Geometry check sheet. Reference: the model listing, model coordinates, mm. A direction names the side the tool comes from. Round coordinates to 2 decimals unless told otherwise and drop trailing zeros. Loops run counter-clockwise (first coordinate to the right, second up) from the corner with the lowest first, then second, coordinate; pieces in that order, holes last. Notation, with made-up numbers: (-15, 35) -> (30, 35) arc R35 ccw to (30, 68) -> close; hole circle Ø4 at (63, 46.5). An arc over 180 degrees is marked (long way). Use a Markdown table: item, result. Add a question column.
Q1. Gauge pin test, flat ends, axial feed: P1, Ø5, axis at x = -1, y = 3.5, coming from the +Z side; P2, Ø1, axis at y = 23, z = 2, coming from the -X side; P3, Ø1.5, axis at y = -12.5, z = 1, coming from the -X side; P4, Ø21, axis at x = 0, y = 0, coming from the +Z side. Record the tip position at first contact, or that the pin passes through.
Q2. Release check for a two-part mould opening along Y. For faces 1 (the face through (-40.786, 1.077, 0.056)), 2 (the face through (-7, 0, -4)), 3 (the face through (-3, -6, -2)) record: released by +Y, released by -Y, zero draft, split by the parting line, or undercut.
Q3. Sectioned sample at A-A, the plane x = 0. Enter the section's corners in (y, z), then the cut area to 3 significant figures.
Q4. Set-up check for faces 4 (the face through (-8.25, -2.6, 0.96)), 5 (the face through (35.252, -0.296, -0.056)): record each of +Z, -Z, +X, -X, +Y, -Y from which the full face is reachable in a straight line by a thin tool's end or side.
Q5. Sectioned sample at B-B, the plane z = -3. Enter the section's corners in (x, y).
Q6. Material ranges on L1, parallel to Y at x = 0, z = -3.45; L2, parallel to Y at x = 20, z = -3; L3, parallel to Y at x = -4.5, z = -2.5, recorded low to high.
Q7. Sectioned sample at C-C, the plane z = 2.25. Enter the section's corners in (x, y), then the cut area to 3 significant figures.
```python
from build123d import *

# Parameters (mm, degrees)
SKETCH_1_R          = 40.8
EXTRUDE_1_DEPTH     = 4
SKETCH_3_R          = 3.15
CUT_EXTRUDE_1_DEPTH = 10
EXTRUDE_START       = -8
EXTRUDE_3_DEPTH     = 8
SKETCH_6_R          = 21
CUT_EXTRUDE_2_DEPTH = 10
SKETCH_7_R          = 0.5
CUT_EXTRUDE_3_DEPTH = 10


with BuildPart() as part:
    # 草图1 → 凸台-拉伸1 (new, symmetric)
    with BuildSketch(Plane.XY):
        Circle(SKETCH_1_R)
    extrude(amount=EXTRUDE_1_DEPTH, both=True)

    # 草图2 → 切除-旋转2 (revolve, cut)
    with BuildSketch(Plane(origin=(0, 0, 0), x_dir=(1, 0, 0), z_dir=(0, 1, 0)), mode=Mode.PRIVATE) as cut_revolve_2_sk:
        Polygon((0, 4), (0, -4), (8.65, -4), (8.65, 2), (6.5, 2), (6.5, 4), align=None)
    revolve(cut_revolve_2_sk.sketch.rotate(Axis((0, 0, -4), (0, 0, 1)), 180), axis=Axis((0, 0, -4), (0, 0, 1)), mode=Mode.SUBTRACT)

    # 草图3 → 切除-旋转3 (revolve, cut)
    with BuildSketch(Plane(origin=(0, 0, 0), x_dir=(1, 0, 0), z_dir=(0, 1, 0))):
        with Locations((31, 5)):
            Circle(SKETCH_3_R)
    revolve(axis=Axis((0, 0, 0), (0, 0, -1)), mode=Mode.SUBTRACT)

    # 草图4 → 切除-拉伸1 (cut)
    with BuildSketch(Plane(origin=(0, 0, -4), x_dir=(-1, 0, 0), z_dir=(0, 0, -1))):
        Polygon((-36, 19.2), (-36, -19.2), (-40.8, -19.2), (-40.8, 0), (-40.8, 19.2), align=None)
    extrude(amount=-CUT_EXTRUDE_1_DEPTH, mode=Mode.SUBTRACT)

    # 草图5 → 凸台-拉伸3 (add)
    with BuildSketch(Plane(origin=(0, 0, -4), x_dir=(-1, 0, 0), z_dir=(0, 0, -1)).offset(EXTRUDE_START)):
        with BuildLine():
            Line((-12.60789337, 38.803105865), (-45, 28.278272418))
            Line((-45, 28.278272418), (-45, -28.278272418))
            Line((-45, -28.278272418), (-12.60789337, -38.803105865))
            ThreePointArc((-12.60789337, -38.803105865), (-24.80809717, -32.391330859), (-34.177392951, -22.283307903))
            Line((-34.177392951, -22.283307903), (-34.876380269, 21.172578948))
            ThreePointArc((-34.876380269, 21.172578948), (-25.32583524, 31.988155142), (-12.60789337, 38.803105865))
        make_face()
    extrude(amount=EXTRUDE_3_DEPTH)

    # 草图6 → 切除-拉伸2 (cut)
    with BuildSketch(Plane(origin=(0, 0, -4), x_dir=(-1, 0, 0), z_dir=(0, 0, -1))):
        with Locations((-56.25, 0)):
            Circle(SKETCH_6_R)
    extrude(amount=-CUT_EXTRUDE_2_DEPTH, mode=Mode.SUBTRACT)

    # 草图7 → 切除-拉伸3 (cut)
    with BuildSketch(Plane(origin=(0, 0, -4), x_dir=(-1, 0, 0), z_dir=(0, 0, -1))):
        with Locations((-42.219558781, 23.005329022)):
            Circle(SKETCH_7_R)
        with Locations((-42.219558781, -23.005329022)):
            Circle(SKETCH_7_R)
        with Locations((37.5, 0)):
            Circle(SKETCH_7_R)
    extrude(amount=-CUT_EXTRUDE_3_DEPTH, mode=Mode.SUBTRACT)


solid = part.part
```
Values:
| question | item | result |
|---|---|---|
| 1 | P1 | through |
| 1 | P2 | x = -34.04 |
| 1 | P3 | x = -39.07 |
| 1 | P4 | z = 4 |
| 2 | face 1 | split by the parting line |
| 2 | face 2 | zero draft |
| 2 | face 3 | undercut |
| 3 | outline | (-40.8, -4) -> (-33.99, -4) arc R3.15 cw to (-28.01, -4) -> (-6.5, -4) -> (-6.5, -2) -> (-8.65, -2) -> (-8.65, 4) -> (-40.8, 4) -> close; (6.5, -4) -> (28.01, -4) arc R3.15 cw to (33.99, -4) -> (40.8, -4) -> (40.8, 4) -> (8.65, 4) -> (8.65, -2) -> (6.5, -2) -> close |
| 3 | area | 504 mm^2 |
| 4 | face 4 | +Z |
| 4 | face 5 | +Z, -Z, +X |
| 5 | outline | circle Ø57.13 at (0, 0); (12.61, -38.8) -> (45, -28.28) -> (45, -17.73) arc R21 cw to (45, 17.73) -> (45, 28.28) -> (12.61, 38.8) arc R40.8 ccw (long way) to start; hole circle Ø1 at (-37.5, 0); hole circle Ø66.87 at (0, 0); hole circle Ø13 at (0, 0); hole circle Ø1 at (42.22, -23.01); hole circle Ø1 at (42.22, 23.01) |
| 6 | L1 | -40.8 to -33.74, -28.26 to -6.5, 6.5 to 28.26, 33.74 to 40.8 |
| 6 | L2 | -36.4 to -26.79, -20.4 to 20.4, 26.79 to 36.4 |
| 6 | L3 | -40.55 to -32.61, -28.73 to -4.69, 4.69 to 28.73, 32.61 to 40.55 |
| 7 | outline | (12.61, -38.8) -> (45, -28.28) -> (45, -17.73) arc R21 cw to (45, 17.73) -> (45, 28.28) -> (12.61, 38.8) arc R40.8 ccw (long way) to start; hole circle Ø1 at (-37.5, 0); hole circle Ø17.3 at (0, 0); hole circle Ø1 at (42.22, -23.01); hole circle Ø1 at (42.22, 23.01) |
| 7 | area | 5,320 mm^2 |
